```python
from build123d import *

# Parameters (mm, degrees)
EXTRUDE1_DEPTH      = 7.9375
EXTRUDE1_DEPTH_BACK = 7.9375
SKETCH2_R           = 1.5875
CHAMFER1_SIZE       = 0.3175


with BuildPart() as part:
    # Sketch2 → Extrude1 (new, two sides: drawn at the far end of the back side and taken through both)
    with BuildSketch(Plane(origin=(0, 0, 0), x_dir=(0, 0, -1), z_dir=(1, 0, 0)).offset(-EXTRUDE1_DEPTH_BACK)):
        Circle(SKETCH2_R)
    extrude(amount=EXTRUDE1_DEPTH + EXTRUDE1_DEPTH_BACK)

    # Chamfer1
    chamfer1_edges = [part.edges().sort_by_distance(p)[0] for p in [
        (-7.9375, 0, 1.5875),
        (7.9375, 0, 1.5875),
    ]]
    chamfer(chamfer1_edges, length=CHAMFER1_SIZE)

    # Sketch3 → Cut-Revolve1 (revolve, cut)
    with BuildSketch(Plane.XY, mode=Mode.PRIVATE) as cut_revolve1_sk:
        with BuildLine():
            Line((3.265089056, 1.5875), (-3.265089056, 1.5875))
            add(Edge.make_bspline(
                [(-3.265089056, 1.5875), (-2.114433092, 1.5875), (-0.878501649, 0.9525), (0, 0.9525)],
                knots=[0, 0, 0, 0, 1, 1, 1, 1], degree=3))
            add(Edge.make_bspline(
                [(3.265089056, 1.5875), (2.114433092, 1.5875), (0.878501649, 0.9525), (0, 0.9525)],
                knots=[0, 0, 0, 0, 1, 1, 1, 1], degree=3))
        make_face()
    revolve(cut_revolve1_sk.sketch.rotate(Axis((7.9375, 0, 0), (-1, 0, 0)), 90), axis=Axis((7.9375, 0, 0), (-1, 0, 0)), mode=Mode.SUBTRACT)


solid = part.part
```
Check sheet for the modelled part. Datum: model origin and axes. Units: mm. Give positions to 0.01 mm unless a question says otherwise; leave off trailing zeros. Loops run counter-clockwise (first coordinate to the right, second up) from the corner with the lowest first, then second, coordinate; pieces in that order, holes last. Notation, with made-up numbers: M 37.25,72 L 47.25,72 A33 ccw 47.25,110 Z; hole C 71,46 d5. An arc over 180 degrees is marked long. Answer as CSV lines item,"result".
Item 1: Depth check by flat-ended pin: pin 1 Ø1.5 at (x, y) = (4.5, 0.5) entering from +Z. Enter the tip coordinate at first touch or a pass-through.
Reply:
pin 1,"z = 1.59"
Item 2: Sectioned sample at A-A, the plane x = -3.75. Enter the section's corners in (y, z) (1 decimal), then the cut area to 3 significant figures.
Reply:
outline,"C 0,0 d3.2"
area,"7.92 mm^2"
Item 3: Draft check along X on faces 1 (the face through (5.41, -1.55, 0.34)), 2 (the face through (7.938, 0, 0)), 3 (the face through (-7.938, 0, 0)). Enter one of: pulls with the +X half, pulls with the -X half, needs draft (parallel to the pull), parting line crosses it, or undercut.
Reply:
face 1,"needs draft"
face 2,"pulls with the +X half"
face 3,"pulls with the -X half"
Item 4: Scan lines: L1, parallel to Y at x = -5.5, z = 0.6; L2, parallel to Z at x = 4.25, y = 1.45; L3, parallel to Z at x = -3.75, y = -0.45. Record each from-to range of solid material in increasing order.
Reply:
L1,"-1.47 to 1.47"
L2,"-0.65 to 0.65"
L3,"-1.52 to 1.52"
